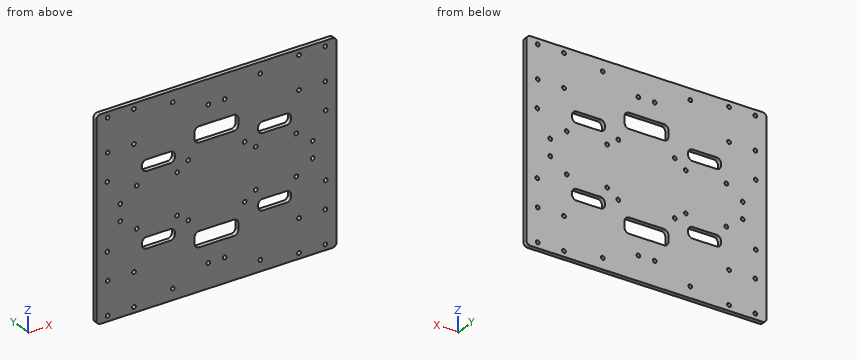
```python
from build123d import *

# Parameters (mm, degrees)
SKETCH_1_W          = 220
SKETCH_1_H          = 180
EXTRUDE_1_DEPTH     = 4
SKETCH_3_R          = 1.75
CUT_EXTRUDE_2_DEPTH = 4
SKETCH_4_R          = 1.75
CUT_EXTRUDE_3_DEPTH = 4
SKETCH_5_R          = 1.75
CUT_EXTRUDE_4_DEPTH = 4
FILLET_1_R          = 4
SKETCH_6_W          = 40
SKETCH_6_H          = 14
SKETCH_6_W_2        = 30
SKETCH_6_H_2        = 10
CUT_EXTRUDE_5_DEPTH = 4
FILLET_2_R          = 4


with BuildPart() as part:
    # 草图1 → 凸台-拉伸1 (new body)
    with BuildSketch(Plane(origin=(0, 0, 0), x_dir=(1, 0, 0), z_dir=(0, 1, 0))):
        Rectangle(SKETCH_1_W, SKETCH_1_H)
    extrude(amount=EXTRUDE_1_DEPTH)

    # 草图3 → 切除-拉伸2 (cut)
    with BuildSketch(Plane.XZ):
        with Locations(Location((-99.5, -55, 0), (0, 0, 270))):
            Circle(SKETCH_3_R)
        with Locations(Location((-75.5, -55, 0), (0, 0, 270))):
            Circle(SKETCH_3_R)
        with Locations(Location((-99.5, -85, 0), (0, 0, 270))):
            Circle(SKETCH_3_R)
        with Locations(Location((-75.5, -85, 0), (0, 0, 270))):
            Circle(SKETCH_3_R)
        with Locations(Location((75.5, -55, 0), (0, 0, 270))):
            Circle(SKETCH_3_R)
        with Locations(Location((99.5, -55, 0), (0, 0, 270))):
            Circle(SKETCH_3_R)
        with Locations(Location((75.5, -85, 0), (0, 0, 270))):
            Circle(SKETCH_3_R)
        with Locations(Location((99.5, -85, 0), (0, 0, 270))):
            Circle(SKETCH_3_R)
        with Locations(Location((-99.5, 85, 0), (0, 0, 270))):
            Circle(SKETCH_3_R)
        with Locations(Location((-75.5, 85, 0), (0, 0, 270))):
            Circle(SKETCH_3_R)
        with Locations(Location((-99.5, 55, 0), (0, 0, 270))):
            Circle(SKETCH_3_R)
        with Locations(Location((-75.5, 55, 0), (0, 0, 270))):
            Circle(SKETCH_3_R)
        with Locations(Location((75.5, 85, 0), (0, 0, 270))):
            Circle(SKETCH_3_R)
        with Locations(Location((99.5, 85, 0), (0, 0, 270))):
            Circle(SKETCH_3_R)
        with Locations(Location((75.5, 55, 0), (0, 0, 270))):
            Circle(SKETCH_3_R)
        with Locations(Location((99.5, 55, 0), (0, 0, 270))):
            Circle(SKETCH_3_R)
        with Locations(Location((-88, 7.5, 0), (0, 0, 270))):
            Circle(SKETCH_3_R)
        with Locations(Location((-88, -7.5, 0), (0, 0, 270))):
            Circle(SKETCH_3_R)
        with Locations(Location((-7.5, -68, 0), (0, 0, 270))):
            Circle(SKETCH_3_R)
        with Locations(Location((7.5, -68, 0), (0, 0, 270))):
            Circle(SKETCH_3_R)
        with Locations(Location((88, -7.5, 0), (0, 0, 270))):
            Circle(SKETCH_3_R)
        with Locations(Location((88, 7.5, 0), (0, 0, 270))):
            Circle(SKETCH_3_R)
        with Locations(Location((-7.5, 68, 0), (0, 0, 270))):
            Circle(SKETCH_3_R)
        with Locations(Location((7.5, 68, 0), (0, 0, 270))):
            Circle(SKETCH_3_R)
    extrude(amount=-CUT_EXTRUDE_2_DEPTH, mode=Mode.SUBTRACT)

    # 草图4 → 切除-拉伸3 (cut)
    with BuildSketch(Plane.XZ):
        with Locations(Location((-73, 18.5, 0), (0, 0, 270))):
            Circle(SKETCH_4_R)
        with Locations(Location((-36, 18.5, 0), (0, 0, 270))):
            Circle(SKETCH_4_R)
        with Locations(Location((-73, -18.5, 0), (0, 0, 270))):
            Circle(SKETCH_4_R)
        with Locations(Location((-36, -18.5, 0), (0, 0, 270))):
            Circle(SKETCH_4_R)
        with Locations(Location((36, 18.5, 0), (0, 0, 270))):
            Circle(SKETCH_4_R)
        with Locations(Location((73, 18.5, 0), (0, 0, 270))):
            Circle(SKETCH_4_R)
        with Locations(Location((36, -18.5, 0), (0, 0, 270))):
            Circle(SKETCH_4_R)
        with Locations(Location((73, -18.5, 0), (0, 0, 270))):
            Circle(SKETCH_4_R)
        with Locations(Location((-25.8, 25.8, 0), (0, 0, 270))):
            Circle(SKETCH_4_R)
        with Locations(Location((25.8, 25.8, 0), (0, 0, 270))):
            Circle(SKETCH_4_R)
        with Locations(Location((-25.8, -25.8, 0), (0, 0, 270))):
            Circle(SKETCH_4_R)
        with Locations(Location((25.8, -25.8, 0), (0, 0, 270))):
            Circle(SKETCH_4_R)
    extrude(amount=-CUT_EXTRUDE_3_DEPTH, mode=Mode.SUBTRACT)

    # 草图5 → 切除-拉伸4 (cut)
    with BuildSketch(Plane.XZ):
        with Locations(Location((-40, 80, 0), (0, 0, 270))):
            Circle(SKETCH_5_R)
        with Locations(Location((40, 80, 0), (0, 0, 270))):
            Circle(SKETCH_5_R)
        with Locations(Location((100, 30, 0), (0, 0, 270))):
            Circle(SKETCH_5_R)
        with Locations(Location((100, -30, 0), (0, 0, 270))):
            Circle(SKETCH_5_R)
        with Locations(Location((40, -80, 0), (0, 0, 270))):
            Circle(SKETCH_5_R)
        with Locations(Location((-40, -80, 0), (0, 0, 270))):
            Circle(SKETCH_5_R)
        with Locations(Location((-100, -30, 0), (0, 0, 270))):
            Circle(SKETCH_5_R)
        with Locations(Location((-100, 30, 0), (0, 0, 270))):
            Circle(SKETCH_5_R)
    extrude(amount=-CUT_EXTRUDE_4_DEPTH, mode=Mode.SUBTRACT)

    # 圆角1
    fillet_1_edges = [part.edges().sort_by_distance(p)[0] for p in [
        (-110, 2, -90),
        (110, 2, -90),
        (110, 2, 90),
        (-110, 2, 90),
    ]]
    fillet(fillet_1_edges, radius=FILLET_1_R)

    # 草图6 → 切除-拉伸5 (cut)
    with BuildSketch(Plane.XZ):
        with Locations((0, 45)):
            Rectangle(SKETCH_6_W, SKETCH_6_H)
        with Locations((-53.094123813, 33.26992324)):
            Rectangle(SKETCH_6_W_2, SKETCH_6_H_2)
        with Locations((53.094123813, 33.26992324)):
            Rectangle(SKETCH_6_W_2, SKETCH_6_H_2)
        with Locations((53.094123813, -33.26992324)):
            Rectangle(SKETCH_6_W_2, SKETCH_6_H_2)
        with Locations((-53.094123813, -33.26992324)):
            Rectangle(SKETCH_6_W_2, SKETCH_6_H_2)
        with Locations((0, -45)):
            Rectangle(SKETCH_6_W, SKETCH_6_H)
    extrude(amount=-CUT_EXTRUDE_5_DEPTH, mode=Mode.SUBTRACT)

    # 圆角2
    fillet_2_edges = [part.edges().sort_by_distance(p)[0] for p in [
        (-38.094123813, 2, 38.26992324),
        (-38.094123813, 2, 28.26992324),
        (-68.094123813, 2, 28.26992324),
        (-68.094123813, 2, 38.26992324),
        (68.094123813, 2, 38.26992324),
        (68.094123813, 2, 28.26992324),
        (38.094123813, 2, 28.26992324),
        (38.094123813, 2, 38.26992324),
        (68.094123813, 2, -28.26992324),
        (68.094123813, 2, -38.26992324),
        (38.094123813, 2, -38.26992324),
        (38.094123813, 2, -28.26992324),
        (-68.094123813, 2, -38.26992324),
        (-68.094123813, 2, -28.26992324),
        (-38.094123813, 2, -28.26992324),
        (-38.094123813, 2, -38.26992324),
        (-20, 2, -52),
        (-20, 2, -38),
        (20, 2, -38),
        (20, 2, -52),
        (20, 2, 52),
        (20, 2, 38),
        (-20, 2, 38),
        (-20, 2, 52),
    ]]
    fillet(fillet_2_edges, radius=FILLET_2_R)


solid = part.part
```
Work out the finished part from the listing and answer in its coordinate system (mm). Round coordinates to 2 decimals unless told otherwise and drop trailing zeros. Order: outer loops, then holes, each group sorted by start corner. A loop starts at its lowest first (then second) coordinate and runs counter-clockwise, first axis right, second up.
Q1. A cutting plane is placed at B-B, the plane y = 1.55. Count the separate pieces of the cut face and the enclosed holes in it, then the cut area to 3 significant figures.
Solution:
separate pieces: 1
enclosed holes: 50
area: 36,900 mm2
Q2. A cutting plane is placed at A-A, the plane x = 51. Determine the outline of the cut face in (y, z).
Solution:
outline: (0, -90) - (4, -90) - (4, -38.27) - (0, -38.27) - close; (0, -28.27) - (4, -28.27) - (4, 28.27) - (0, 28.27) - close; (0, 38.27) - (4, 38.27) - (4, 90) - (0, 90) - close
Q3. Find the intervals of material crossed by line 1 along X through (y, z) = (1.5, 68); line 2 along X through (y, z) = (2.6, -80); line 3 along Z through (x, y) = (-9.5, 0.9), in increasing order.
Solution:
line 1: x = -110 to -9.25, -5.75 to 5.75, 9.25 to 110
line 2: x = -110 to -41.75, -38.25 to 38.25, 41.75 to 110
line 3: z = -90 to -52, -38 to 38, 52 to 90
